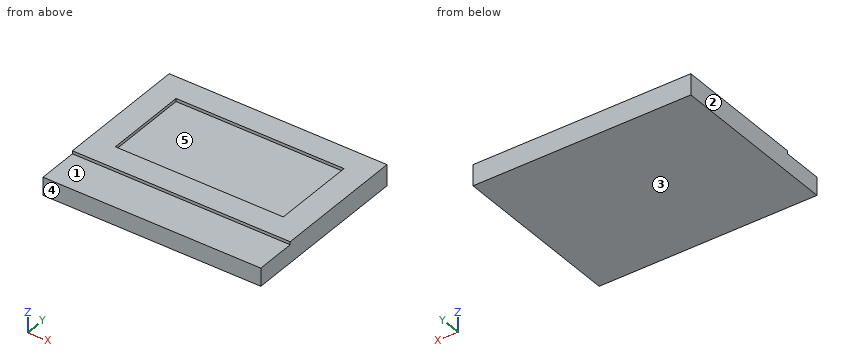
```python
from build123d import *

# Parameters (mm, degrees)
SKETCH1_W           = 145
SKETCH1_H           = 116
BOSS_EXTRUDE1_DEPTH = 12
SKETCH2_W           = 145
SKETCH2_H           = 89
SKETCH2_W_2         = 111.8
SKETCH2_H_2         = 55.8
BOSS_EXTRUDE2_DEPTH = 2


with BuildPart() as part:
    # Sketch1 → Boss-Extrude1 (new body)
    with BuildSketch(Plane.XY):
        Rectangle(SKETCH1_W, SKETCH1_H)
    extrude(amount=BOSS_EXTRUDE1_DEPTH)

    # Sketch2 → Boss-Extrude2 (add)
    with BuildSketch(Plane.XY.offset(12)):
        with Locations((0, 13.5)):
            Rectangle(SKETCH2_W, SKETCH2_H)
        with Locations((0, 13.5)):
            Rectangle(SKETCH2_W_2, SKETCH2_H_2, mode=Mode.SUBTRACT)
    extrude(amount=BOSS_EXTRUDE2_DEPTH)


solid = part.part
```
Design review of the part built by this model. Coordinates are the model's own, in mm. Face numbers are marked on the shaded views. A direction names the side the tool comes from. Give positions to 0.01 mm unless a question says otherwise; leave off trailing zeros. Loops run counter-clockwise (first coordinate to the right, second up) from the corner with the lowest first, then second, coordinate; pieces in that order, holes last. Notation, with made-up numbers: (84, 12) -> (134, 12) arc R21 ccw to (134, 24) -> close; hole circle Ø8 at (-19, -3.75). An arc over 180 degrees is marked (long way). One line per item, written item: value.
Q1. We need section B-B on x = 3.5. Give the boundary of the cut face in (y, z).
Numbers:
outline: (-58, 0) -> (58, 0) -> (58, 14) -> (41.4, 14) -> (41.4, 12) -> (-14.4, 12) -> (-14.4, 14) -> (-31, 14) -> (-31, 12) -> (-58, 12) -> close
Q2. For L1, parallel to Y at x = 25.5, z = 13; L2, parallel to X at y = 1.5, z = 12.5; L3, parallel to Z at x = 39, y = -33.5, list the stretches that pass through material, from the lowest coordinate up.
Numbers:
L1: y = -31 to -14.4, 41.4 to 58
L2: x = -72.5 to -55.9, 55.9 to 72.5
L3: z = 0 to 12
Q3. Machinability: for the marked faces 1 and 2, which of the approach directions +Z, -Z, +X, -X, +Y, -Y give a long, thin tool a straight path to every point of the face, cutting with its end or side? Answer none if there is none.
Numbers:
face 1: +Z, +X, -X, -Y
face 2: +Z, -Z, -X, +Y, -Y
Q4. We need section A-A on y = -4.5. Give the boundary of the cut face in (x, z).
Numbers:
outline: (-72.5, 0) -> (72.5, 0) -> (72.5, 14) -> (55.9, 14) -> (55.9, 12) -> (-55.9, 12) -> (-55.9, 14) -> (-72.5, 14) -> close
Q5. For pin 1 Ø3 at (x, y) = (-14.5, 3) entering from +Z; pin 2 Ø8 at (x, y) = (-52, -30.5) entering from -Z; pin 3 Ø0.6 at (x, z) = (-13.5, 12.5) entering from -Y, all flat-tipped, find the tip position at first contact; note any pin that passes through.
Numbers:
pin 1: stops at z = 12
pin 2: stops at z = 0
pin 3: stops at y = -31
Q6. Draft analysis for pull direction Y (two halves, no side actions). For the marked faces 3, 4 and 5, state which applies: pulls with the +Y half, pulls with the -Y half, needs draft (parallel to the pull), parting line crosses it, or undercut.
Numbers:
face 3: needs draft
face 4: pulls with the -Y half
face 5: undercut
